Geometry check sheet. Reference: the model listing, model coordinates, mm. Face numbers are marked on the shaded views. Give positions to 0.01 mm unless a question says otherwise; leave off trailing zeros. Write each loop counter-clockwise with the first axis right and the second up, starting at its lowest first coordinate (ties: lowest second). Pieces come first, ordered by that corner, then holes. Notation, with made-up numbers: (27, -39) -> (45, -39) arc R29 ccw to (45, -9) -> close; hole circle Ø1 at (25, 79.5). An arc over 180 degrees is marked (long way). Use a Markdown table: item, result. Add a question column.
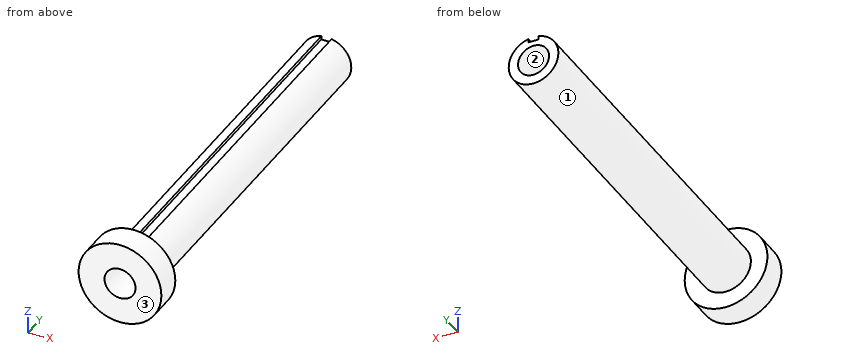
from build123d import *

# Parameters (mm, degrees)
SKETCH1_R               = 6.096
SKETCH1_R_2             = 3.81
BOSS_EXTRUDE1_DEPTH     = 97.79
SKETCH2_W               = 2.54
SKETCH2_H               = 1.627681679
CUT_EXTRUDE1_DEPTH      = 1
CUT_EXTRUDE1_DEPTH_BACK = 98.79
SKETCH3_R               = 10.16
SKETCH3_R_2             = 3.81
BOSS_EXTRUDE2_DEPTH     = 6.604


with BuildPart() as part:
    # Sketch1 → Boss-Extrude1 (new body)
    with BuildSketch(Plane(origin=(0, 0, 0), x_dir=(1, 0, 0), z_dir=(0, 1, 0))):
        Circle(SKETCH1_R)
        Circle(SKETCH1_R_2, mode=Mode.SUBTRACT)
    extrude(amount=BOSS_EXTRUDE1_DEPTH)

    # Sketch2 → Cut-Extrude1 (cut, two sides)
    with BuildSketch(Plane.XZ) as cut_extrude1_sk:
        with Locations((0, 5.89384084)):
            Rectangle(SKETCH2_W, SKETCH2_H)
    extrude(amount=CUT_EXTRUDE1_DEPTH, mode=Mode.SUBTRACT)
    extrude(cut_extrude1_sk.sketch, amount=-CUT_EXTRUDE1_DEPTH_BACK, mode=Mode.SUBTRACT)

    # Sketch3 → Boss-Extrude2 (add)
    with BuildSketch(Plane.XZ):
        Circle(SKETCH3_R)
        Circle(SKETCH3_R_2, mode=Mode.SUBTRACT)
    extrude(amount=-BOSS_EXTRUDE2_DEPTH)


solid = part.part
1) Sectioned sample at D-D, the plane z = -8. Enter the section's corners in (x, y).
2) Gauge pin test, flat ends, axial feed: P1, Ø3, axis at x = -0.5, y = 63.5, coming from the +Z side; P2, Ø6, axis at x = -0.5, y = 82.5, coming from the -Z side; P3, Ø8, axis at y = 52, z = 3.5, coming from the +X side; P4, Ø3, axis at x = -4.5, z = -3, coming from the -Y side. Record the tip position at first contact, or that the pin passes through.
3) Sectioned sample at A-A, the plane z = 0. Enter the section's corners in (x, y).
4) Sectioned sample at B-B, the plane x = 0. Enter the section's corners in (y, z), and give its area (3 significant figures).
5) Material ranges on probe 1 along X at (y, z) = (31, 0); probe 2 along Y at (x, z) = (6.25, -5.5); probe 3 along Z at (x, y) = (4.75, 69.5), recorded low to high. Write a range as [from, to].
6) Sectioned sample at C-C, the plane y = 44. Enter the section's corners in (x, z).
7) Draft check along Z on the marked faces 1, 2 and 3. Enter one of: +Z half, -Z half, draft (parallel to the pull), parting line (faces both ways), or undercut.
Check values:
| question | item | result |
|---|---|---|
| 1 | outline | (-6.26, 0) -> (6.26, 0) -> (6.26, 6.6) -> (-6.26, 6.6) -> close |
| 2 | P1 | z = 5.96 |
| 2 | P2 | z = -6.1 |
| 2 | P3 | x = 6.1 |
| 2 | P4 | y = 0 |
| 3 | outline | (-10.16, 0) -> (-3.81, 0) -> (-3.81, 97.79) -> (-6.1, 97.79) -> (-6.1, 6.6) -> (-10.16, 6.6) -> close; (3.81, 0) -> (10.16, 0) -> (10.16, 6.6) -> (6.1, 6.6) -> (6.1, 97.79) -> (3.81, 97.79) -> close |
| 4 | outline | (0, -10.16) -> (6.6, -10.16) -> (6.6, -6.1) -> (97.79, -6.1) -> (97.79, -3.81) -> (0, -3.81) -> close; (0, 3.81) -> (97.79, 3.81) -> (97.79, 5.08) -> (6.6, 5.08) -> (6.6, 10.16) -> (0, 10.16) -> close |
| 4 | area | 408 mm² |
| 5 | probe 1 | [-6.1, -3.81], [3.81, 6.1] |
| 5 | probe 2 | [0, 6.6] |
| 5 | probe 3 | [-3.82, 3.82] |
| 6 | outline | (-1.27, 5.08) -> (-1.27, 5.96) arc R6.1 ccw (long way) to (1.27, 5.96) -> (1.27, 5.08) -> close; hole circle Ø7.62 at (0, 0) |
| 7 | face 1 | parting line |
| 7 | face 2 | undercut |
| 7 | face 3 | draft |
